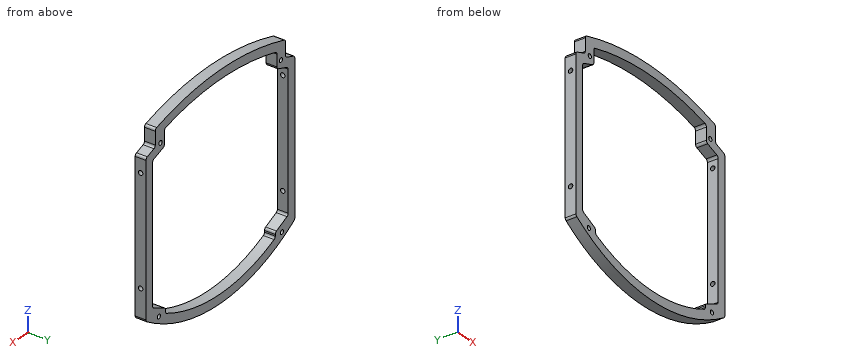
```python
from build123d import *

# Parameters (mm, degrees)
SKETCH1_R                        = 1.2
BOSS_EXTRUDE1_DEPTH              = 6
TAP_DRILL_FOR_M3_TAP1_AT_2_COUNT = 2
TAP_DRILL_FOR_M3_TAP1_AT_2_PITCH = 60
FILLET1_R                        = 1.5


with BuildPart() as part:
    # Sketch1 → Boss-Extrude1 (new body)
    with BuildSketch(Plane(origin=(0, 0, 0), x_dir=(1, 0, 0), z_dir=(0, 1, 0))):
        with BuildLine():
            Line((-56, -46.878887336), (-56, 38))
            ThreePointArc((-56, 38), (0, 55.150739291), (56, 38))
            Line((56, 38), (56, -46.696902219))
            Line((56, -46.696902219), (49, -49.244693859))
            Line((49, -49.244693859), (49, -58.574358685))
            ThreePointArc((49, -58.574358685), (0, -66.262179264), (-49, -58.574358685))
            Line((-49, -58.574358685), (-49, -49.426678976))
            Line((-49, -49.426678976), (-56, -46.878887336))
        make_face()
        with Locations((-46.3, 40)):
            Circle(SKETCH1_R, mode=Mode.SUBTRACT)
        with Locations((46.3, 40)):
            Circle(SKETCH1_R, mode=Mode.SUBTRACT)
        with Locations((45.1, -49.6)):
            Circle(SKETCH1_R, mode=Mode.SUBTRACT)
        with Locations((-45.6, -49.6)):
            Circle(SKETCH1_R, mode=Mode.SUBTRACT)
        with BuildLine():
            Line((-51, -43.377849645), (-51, 33.394842331))
            Line((-51, 33.394842331), (-41.3, 37.918026615))
            Line((-41.3, 37.918026615), (-41.3, 40.703705341))
            ThreePointArc((-41.3, 40.703705341), (0, 50.150739291), (41.3, 40.703705341))
            Line((41.3, 40.703705341), (41.3, 37.918026615))
            Line((41.3, 37.918026615), (51, 33.394842331))
            Line((51, 33.394842331), (51, -43.195864528))
            Line((51, -43.195864528), (42.1, -46.435199613))
            Line((42.1, -46.435199613), (42.1, -55.435199613))
            ThreePointArc((42.1, -55.435199613), (-0.259888817, -61.261961386), (-42.6, -55.29318275))
            Line((-42.6, -55.29318275), (-42.6, -46.435199613))
            Line((-42.6, -46.435199613), (-51, -43.377849645))
        make_face(mode=Mode.SUBTRACT)
    extrude(amount=BOSS_EXTRUDE1_DEPTH)

    # Sketch2 → Tap Drill for M3 Tap1 (revolve, cut)
    with BuildSketch(Plane(origin=(-56, 3, -21.857868774), x_dir=(0, 0, 1), z_dir=(0, 1, 0))):
        Polygon((0, 0), (0, 10.751075774), (1.25, 10), (1.25, 0), align=None)
    tap_drill_for_m3_tap1 = revolve(axis=Axis((-62.35, 3, -21.857868774), (1, 0, 0)), mode=Mode.SUBTRACT)

    # Tap Drill for M3 Tap1 at 2: Tap Drill for M3 Tap1 ×2
    with Locations(*[(0, 0, i * TAP_DRILL_FOR_M3_TAP1_AT_2_PITCH) for i in range(1, TAP_DRILL_FOR_M3_TAP1_AT_2_COUNT)]):
        add(tap_drill_for_m3_tap1, mode=Mode.SUBTRACT)

    # Mirror1: Tap Drill for M3 Tap1 across plane
    add(tap_drill_for_m3_tap1.mirror(Plane(origin=(0, 0, 0), x_dir=(0, 0, 1), z_dir=(1, 0, 0))), mode=Mode.SUBTRACT)

    # Mirror1 copy 1 sketch → Mirror1 copy 1 (revolve, cut)
    with BuildSketch(Plane(origin=(56, 3, 38.142131226), x_dir=(0, 0, 1), z_dir=(0, 1, 0))):
        Polygon((0, 0), (0, -10.751075774), (1.25, -10), (1.25, 0), align=None)
    revolve(axis=Axis((62.35, 3, 38.142131226), (1, 0, 0)), mode=Mode.SUBTRACT)

    # Fillet1
    fillet1_edges = [part.edges().sort_by_distance(p)[0] for p in [
        (49, 3, 49.244693859),
        (49, 3, 58.574358685),
        (-49, 3, 58.574358685),
        (-49, 3, 49.426678976),
        (-56, 3, 46.878887336),
        (-56, 3, -38),
        (56, 3, -38),
        (56, 3, 46.696902219),
        (-51, 3, 43.377849645),
        (-42.6, 3, 46.435199613),
        (-42.6, 3, 55.29318275),
        (42.1, 3, 55.435199613),
        (42.1, 3, 46.435199613),
        (51, 3, 43.195864528),
        (51, 3, -33.394842331),
        (41.3, 3, -37.918026615),
        (41.3, 3, -40.703705341),
        (-41.3, 3, -40.703705341),
        (-41.3, 3, -37.918026615),
        (-51, 3, -33.394842331),
    ]]
    fillet(fillet1_edges, radius=FILLET1_R)


solid = part.part
```
Here's how the part is built. I have some questions about the finished solid (model axes, mm). Round coordinates to 2 decimals unless told otherwise and drop trailing zeros. Loops run counter-clockwise (first coordinate to the right, second up) from the corner with the lowest first, then second, coordinate; pieces in that order, holes last. Notation, with made-up numbers: (-2, 79.25) -> (27, 79.25) arc R7 ccw to (27, 89.25) -> close; hole circle Ø1 at (62.5, 17.25). An arc over 180 degrees is marked (long way). Answer as CSV lines item,"result".
1. If I drill on L1, parallel to Z at x = -45.6, y = 3.75; L2, parallel to Z at x = 52.45, y = 3; L3, parallel to X at y = 5, z = -21, over which ranges is the centre line in solid material (lowest first)?
Final values:
L1,"z = -44.15 to -40.97, -39.03 to -35.91, 45.34 to 48.4, 50.8 to 59.63"
L2,"z = -40.29 to -23.11, -20.61 to 36.89, 39.39 to 47.99"
L3,"x = -56 to -51, 51 to 56"
2. For pin 1 (1 mm diameter, centred on y = 3.5, z = -39.5, fed in from -X); pin 2 (1.5 mm diameter, centred on y = 4.5, z = 46.5, fed in from +X); pin 3 (2 mm diameter, centred on y = 3, z = 38.14, fed in from +X); pin 4 (3 mm diameter, centred on y = 2.5, z = 55, fed in from +X), each with a flat end and sliding along its axis, tell me the tip position at first contact or that it passes through.
Final values:
pin 1,"stops at x = -54.49"
pin 2,"stops at x = 56"
pin 3,"passes through"
pin 4,"stops at x = 49"
3. If we section it at C-C on y = 3: Count the separate pieces of the cut face and the enclosed holes in it, plus the area to 3 significant figures.
Final values:
separate pieces,"4"
enclosed holes,"4"
area,"2,030 mm^2"
4. If we section it at A-A on z = -18: Please give me the cut outline in (x, y), plus the area to 3 significant figures.
Final values:
outline,"(-56, 0) -> (-51, 0) -> (-51, 6) -> (-56, 6) -> close; (51, 0) -> (56, 0) -> (56, 6) -> (51, 6) -> close"
area,"60.0 mm^2"
5. If we section it at B-B on x = 4: Please give me the cut outline in (y, z).
Final values:
outline,"(0, -55.07) -> (6, -55.07) -> (6, -50.07) -> (0, -50.07) -> close; (0, 61.21) -> (6, 61.21) -> (6, 66.21) -> (0, 66.21) -> close"
